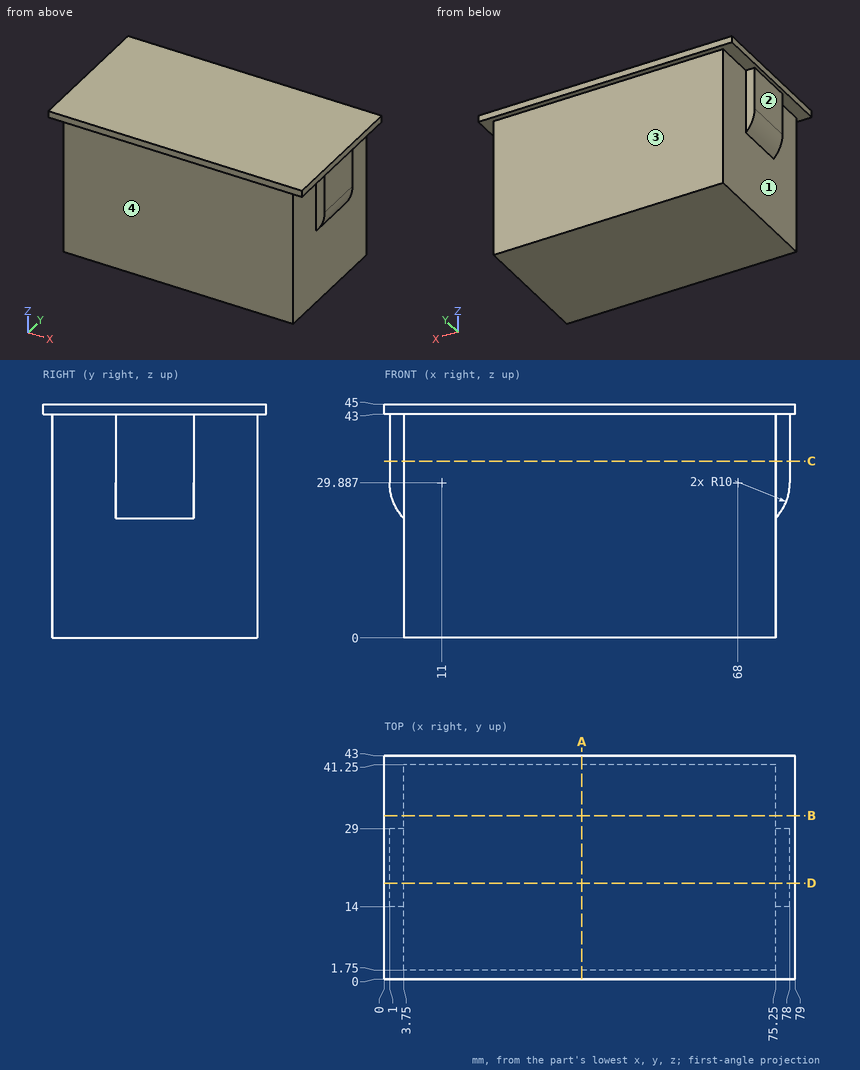
Print and shaded views of the part. All mm, measured from the part's lowest x, y and z. A direction names the side the tool comes from. Round coordinates to 2 decimals unless told otherwise and drop trailing zeros. Write each loop counter-clockwise with the first axis right and the second up, starting at its lowest first coordinate (ties: lowest second). Pieces come first, ordered by that corner, then holes. Notation, with made-up numbers: M 78.5,36 L 106.5,36 A16 cw 106.5,66 Z; hole C 52,-6.75 d11. An arc over 180 degrees is marked long. One line per question, with ' | ' between items.
(1) Saw through at C-C on z = 34. Write the cut outline in (x, y), then the cut area to 3 significant figures.
Answer key:
outline: M 1,14 L 3.75,14 L 3.75,1.75 L 75.25,1.75 L 75.25,14 L 78,14 L 78,29 L 75.25,29 L 75.25,41.25 L 3.75,41.25 L 3.75,29 L 1,29 Z | area: 2,910 mm^2
(2) 3-axis set-ups, long thin cutter, end or side, ignore diameter. For the marked faces 1, 2, 3 and 4: which of +Z, -Z, +X, -X, +Y, -Y reach the whole face in a straight line?
Answer key:
face 1: -Z, -X | face 2: -Z, -X, +Y, -Y | face 3: -Z, +X, -X, +Y | face 4: -Z, +X, -X, -Y
(3) Pin check, flat tips, straight feed: pin 1 (5 mm diameter, centred on x = 65, z = 23, fed in from -Y); pin 2 (2 mm diameter, centred on x = 2.5, z = 32, fed in from +Y); pin 3 (20 mm diameter, centred on y = 27, z = 24, fed in from +X). Stop position of each tip, or through.
Answer key:
pin 1: stops at y = 1.75 | pin 2: stops at y = 29 | pin 3: stops at x = 78
(4) Saw through at A-A on x = 38. Write the cut outline in (y, z).
Answer key:
outline: M 0,43 L 1.75,43 L 1.75,0 L 41.25,0 L 41.25,43 L 43,43 L 43,45 L 0,45 Z
(5) Saw through at D-D on y = 18.5. Write the cut outline in (x, z), then the cut area to 3 significant figures.
Answer key:
outline: M 0,43 L 1,43 L 1,29.89 A10 ccw 3.75,23 L 3.75,0 L 75.25,0 L 75.25,23 A10 ccw 78,29.89 L 78,43 L 79,43 L 79,45 L 0,45 Z | area: 3,330 mm^2
(6) Probe line 1 along Y through (x, z) = (4, 22); line 2 along X through (y, z) = (17.5, 11); line 3 along X through (y, z) = (23.5, 29). List the from-to ranges inside material, lowest first.
Answer key:
line 1: y = 1.75 to 41.25 | line 2: x = 3.75 to 75.25 | line 3: x = 1.04 to 77.96
(7) Saw through at B-B on y = 31.5. Write the cut outline in (x, z), then the cut area to 3 significant figures.
Answer key:
outline: M 0,43 L 3.75,43 L 3.75,0 L 75.25,0 L 75.25,43 L 79,43 L 79,45 L 0,45 Z | area: 3,230 mm^2
